The drawing under review shows one solid part. Ordinate dimensions are in mm from its lowest x, y, z. Round coordinates to 2 decimals unless told otherwise and drop trailing zeros. Loops run counter-clockwise (first coordinate to the right, second up) from the corner with the lowest first, then second, coordinate; pieces in that order, holes last. Notation, with made-up numbers: (-18, 68) - (15, 68) arc R24 ccw to (15, 107) - close; hole circle Ø7 at (85.25, 38.25). An arc over 180 degrees is marked (long way). Answer as CSV lines item,"result".
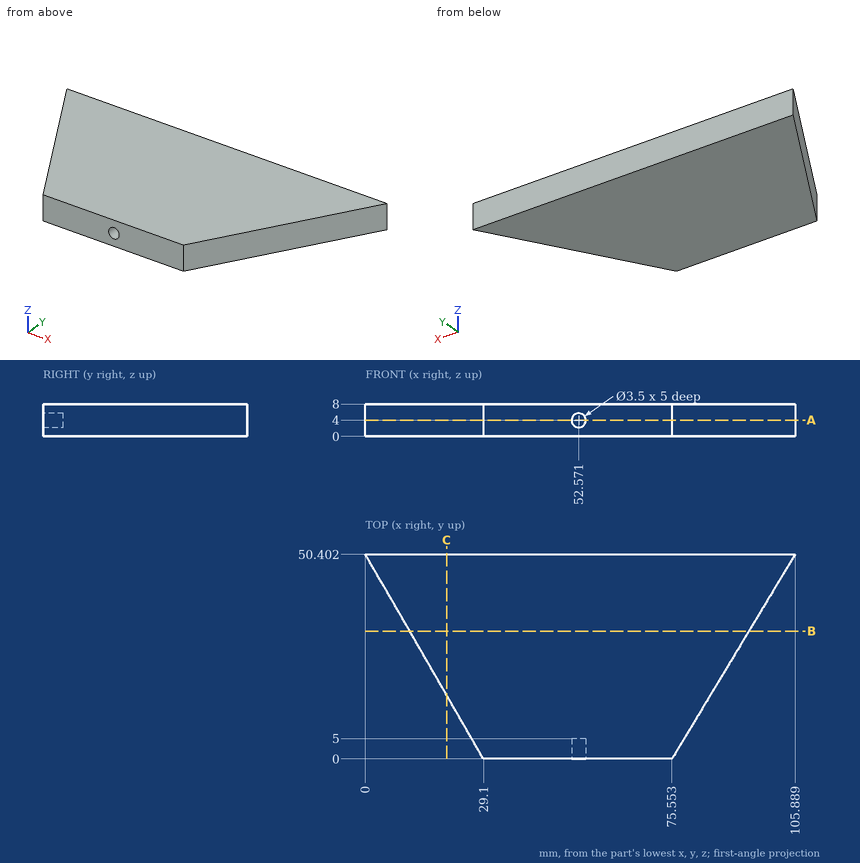
1. Take a section at A-A (z = 4). State the section outline as (x, y) points.
Numbers:
outline,"(0, 50.4) - (29.1, 0) - (50.82, 0) - (50.82, 5) - (54.32, 5) - (54.32, 0) - (75.55, 0) - (105.89, 50.4) - close"
2. Take a section at C-C (x = 20). State the section outline as (y, z) points.
Numbers:
outline,"(15.76, 0) - (50.4, 0) - (50.4, 8) - (15.76, 8) - close"
3. Take a section at B-B (y = 31.5). State the section outline as (x, z) points, plus the area to 3 significant figures.
Numbers:
outline,"(10.91, 0) - (94.51, 0) - (94.51, 8) - (10.91, 8) - close"
area,"669 mm²"
4. Clearance check with flat-ended pins moving along their axes: pin 1 (1.5 mm diameter, centred on y = 38.5, z = 2, fed in from -X); pin 2 (1 mm diameter, centred on x = 52.5, z = 4.5, fed in from -Y); pin 3 (4 mm diameter, centred on y = 36.5, z = 5.5, fed in from -X). State where each tip first meets the part, or that it passes through.
Numbers:
pin 1,"stops at x = 6.44"
pin 2,"stops at y = 5"
pin 3,"stops at x = 6.87"
5. Wall thickness on probe 1 along X at (y, z) = (3.5, 4); probe 2 along X at (y, z) = (2.3, 4) (1 decimal); probe 3 along Y at (x, z) = (53.5, 3): over which ranges is each line inside the solid? List them lowest first.
Numbers:
probe 1,"x = 27.08 to 50.82, 54.32 to 77.66"
probe 2,"x = 27.8 to 50.8, 54.3 to 76.9"
probe 3,"y = 5 to 50.4"
